Read the model definition and answer for the solid it produces. Units are mm, in the model's axes. A direction names the side the tool comes from. Coordinates: 2 decimals unless noted, no trailing zeros. Write each loop counter-clockwise with the first axis right and the second up, starting at its lowest first coordinate (ties: lowest second). Pieces come first, ordered by that corner, then holes.
1) Determine the mould class of faces 1 (the face through (16, 12.7, -1)), 2 (the face through (-30.235, 6.261, 23.183)), 3 (the face through (-2.381, 8, 25)) for opening direction X: +X half, -X half, draft (parallel to the pull), parting line (faces both ways), or undercut.
2) The part is cut by section B-B (z = 2.5). Determine the outline of the cut face in (x, y) (3 decimals), then the cut area to 3 significant figures.
3) Find the intervals of material crossed by line 1 (X direction, y = 5.5, z = 0); line 2 (X direction, y = 8.5, z = 24); line 3 (Y direction, x = -10.5, z = 4) (3 decimals), in increasing order.
4) The part is cut by section D-D (x = -17). Determine the outline of the cut face in (y, z).
5) The part is cut by section A-A (x = 0). Determine the outline of the cut face in (y, z) (3 decimals).
6) The part is cut by section C-C (y = 11). Determine the outline of the cut face in (x, z), then the cut area to 3 significant figures.
7) Which of the six approach directions +Z, -Z, +X, -X, +Y, -Y give full straight-line access (tool end or side, diameter ignored) to faces 4 (the face through (2.381, 8, 25)), 5 (the face through (-1, 0, -1)), 6 (the face through (0.53, 8, -12.72))?
8) Each of these flat-tipped pins is pushed along its axis until it touches: pin 1 Ø23 at (x, z) = (0, 0) entering from -Y; pin 2 Ø1 at (x, y) = (-16, 8) entering from +Z; pin 3 Ø3 at (y, z) = (7, 27) entering from -X; pin 4 Ø1 at (y, z) = (5, 12) entering from +X. Where does it stop, or does it pass through?
from build123d import *

# Parameters (mm, degrees)
SKETCH1_R           = 38.1
BOSS_EXTRUDE1_DEPTH = 12.7
CUT_EXTRUDE1_DEPTH  = 9.525


with BuildPart() as part:
    # Sketch1 → Boss-Extrude1 (new body)
    with BuildSketch(Plane(origin=(0, 0, 0), x_dir=(1, 0, 0), z_dir=(0, 1, 0))):
        Circle(SKETCH1_R)
    extrude(amount=BOSS_EXTRUDE1_DEPTH)

    # Sketch2 → Cut-Extrude1 (cut)
    with BuildSketch(Plane(origin=(0, 12.7, 0), x_dir=(1, 0, 0), z_dir=(0, 1, 0))):
        with BuildLine():
            Line((2.38125, -38.025513125), (2.38125, -12.507082254))
            ThreePointArc((2.38125, -12.507082254), (0, 12.73175), (-2.38125, -12.507082254))
            Line((-2.38125, -12.507082254), (-2.38125, -38.025513125))
            ThreePointArc((-2.38125, -38.025513125), (0, -38.1), (2.38125, -38.025513125))
        make_face()
    extrude(amount=-CUT_EXTRUDE1_DEPTH, mode=Mode.SUBTRACT)


solid = part.part
Reported:
1. face 1: draft
1. face 2: parting line
1. face 3: undercut
2. outline: (-38.018, 0) - (38.018, 0) - (38.018, 12.7) - (12.484, 12.7) - (12.484, 3.175) - (-12.484, 3.175) - (-12.484, 12.7) - (-38.018, 12.7) - close
2. area: 728 mm2
3. line 1: x = -38.1 to -12.73, 12.73 to 38.1
3. line 2: x = -29.59 to -2.38, 2.38 to 29.59
3. line 3: y = 0 to 3.175
4. outline: (0, -34.1) - (12.7, -34.1) - (12.7, 34.1) - (0, 34.1) - close
5. outline: (0, -38.1) - (12.7, -38.1) - (12.7, -12.732) - (3.175, -12.732) - (3.175, 38.1) - (0, 38.1) - close
6. outline: (-2.38, 12.51) - (-2.38, 38.03) arc R38.1 ccw (long way) to (2.38, 38.03) - (2.38, 12.51) arc R12.73 cw (long way) to start
6. area: 3,930 mm2
7. face 4: +Z, +Y
7. face 5: +Z, -Z, +X, -X, -Y
7. face 6: +Y
8. pin 1: stops at y = 0
8. pin 2: stops at z = 34.8
8. pin 3: stops at x = -28.31
8. pin 4: stops at x = 36.32
